The figure shows three views and two pictorial views of one solid part (mm, origin at its lowest corner). Answer the questions. Coordinates: 2 decimals unless noted, no trailing zeros. Loops run counter-clockwise (first coordinate to the right, second up) from the corner with the lowest first, then second, coordinate; pieces in that order, holes last.
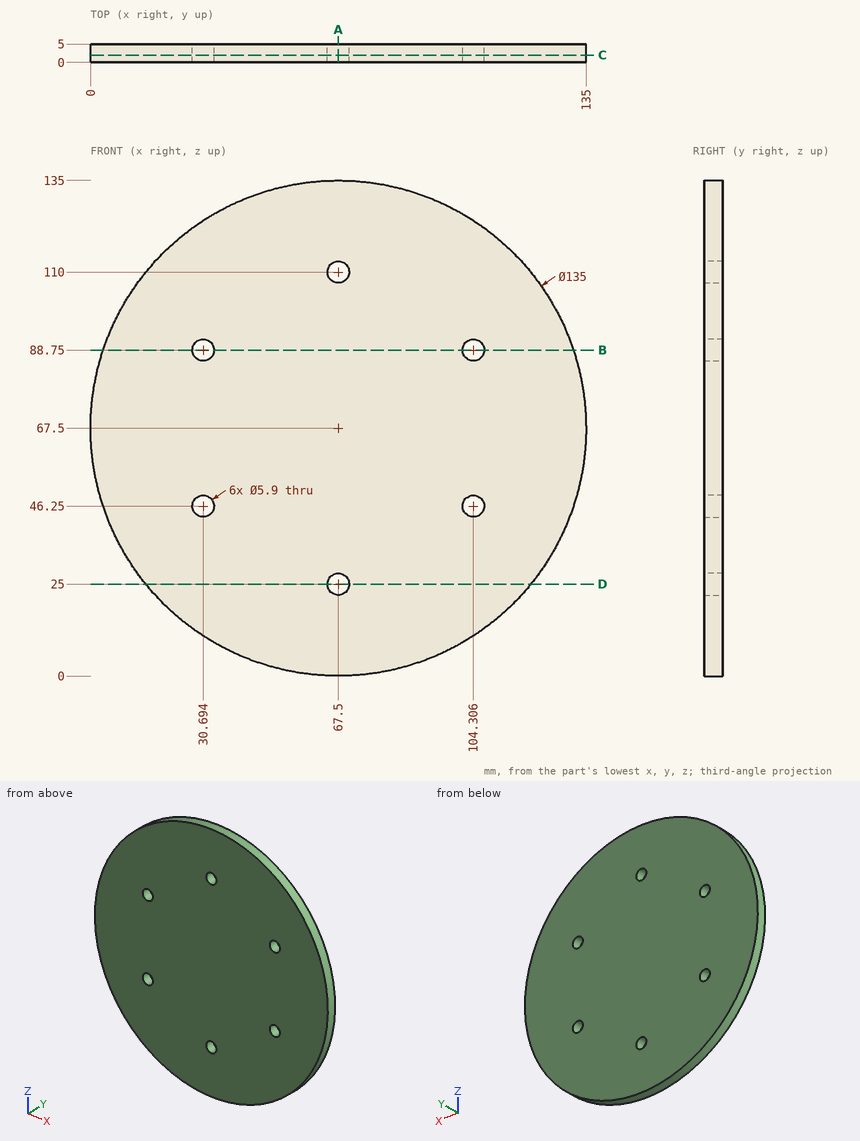
Q1. A cutting plane is placed at D-D (z = 25). Give the vertices of the cut face in (x, y).
Findings below:
outline: (15.06, 0) - (64.55, 0) - (64.55, 5) - (15.06, 5) - close; (70.45, 0) - (119.94, 0) - (119.94, 5) - (70.45, 5) - close
Q2. A cutting plane is placed at C-C (y = 1.95). Give the vertices of the cut face in (x, z).
Findings below:
outline: circle Ø135 at (67.5, 67.5); hole circle Ø5.9 at (30.69, 46.25); hole circle Ø5.9 at (30.69, 88.75); hole circle Ø5.9 at (67.5, 25); hole circle Ø5.9 at (67.5, 110); hole circle Ø5.9 at (104.31, 46.25); hole circle Ø5.9 at (104.31, 88.75)
Q3. Flat-ended cylindrical pins translate along their axes: pin 1 Ø1.5 at (x, y) = (118.5, 0.5) entering from -Z; pin 2 Ø3 at (x, y) = (112.5, 4) entering from +Z; pin 3 Ø3 at (x, y) = (33.5, 3) entering from +Z. Find the tip coordinate at first contact, or state that the pin passes through.
Findings below:
pin 1: stops at z = 22.43
pin 2: stops at z = 119.11
pin 3: stops at z = 126.66
Q4. Straight lines are drawn through the part: probe 1 along X at (y, z) = (2.65, 88.75); probe 2 along X at (y, z) = (3.75, 65.5); probe 3 along Z at (x, y) = (105.5, 0.5). For each, find the intervals that lie inside material, in ascending order.
Findings below:
probe 1: x = 3.43 to 27.74, 33.64 to 101.36, 107.26 to 131.57
probe 2: x = 0.03 to 134.97
probe 3: z = 11.71 to 43.55, 48.95 to 86.05, 91.45 to 123.29
Q5. A cutting plane is placed at A-A (x = 67.5). Give the vertices of the cut face in (y, z), then the cut area to 3 significant figures.
Findings below:
outline: (0, 0) - (5, 0) - (5, 22.05) - (0, 22.05) - close; (0, 27.95) - (5, 27.95) - (5, 107.05) - (0, 107.05) - close; (0, 112.95) - (5, 112.95) - (5, 135) - (0, 135) - close
area: 616 mm2
Q6. A cutting plane is placed at B-B (z = 88.75). Give the vertices of the cut face in (x, y).
Findings below:
outline: (3.43, 0) - (27.74, 0) - (27.74, 5) - (3.43, 5) - close; (33.64, 0) - (101.36, 0) - (101.36, 5) - (33.64, 5) - close; (107.26, 0) - (131.57, 0) - (131.57, 5) - (107.26, 5) - close
